For this review, take the finished solid that the model builds, in its own axes (mm). Coordinates: 2 decimals unless noted, no trailing zeros. Write each loop counter-clockwise with the first axis right and the second up, starting at its lowest first coordinate (ties: lowest second). Pieces come first, ordered by that corner, then holes.
1) We need section A-A on z = 289.5. Write out the cut boundary in (x, y).
2) To check wall thickness, follow line 1 along Z through (x, y) = (146.5, -148.5); line 2 along X through (y, z) = (301, 546); line 3 along X through (y, z) = (57, 558.5). State the ranges of each line that lie inside material, in increasing order.
3) Insertion check: P1, Ø25, axis at y = -366.5, z = 110.5, coming from the -X side; P2, Ø10, axis at x = -10, y = -285, coming from the -Z side; P3, Ø8, axis at x = -138.5, y = 116, coming from the +Z side. Each pin has a flat end and moves straight along its axis. Give the tip position at first contact, or say it passes through.
4) We need section C-C on y = -138. Write out the cut boundary in (x, z), then the cut area to 3 significant figures.
5) We need section B-B on y = 24. Write out the cut boundary in (x, z), then the cut area to 3 significant figures.
6) We need section D-D on x = 92.5. Write out the cut boundary in (y, z).
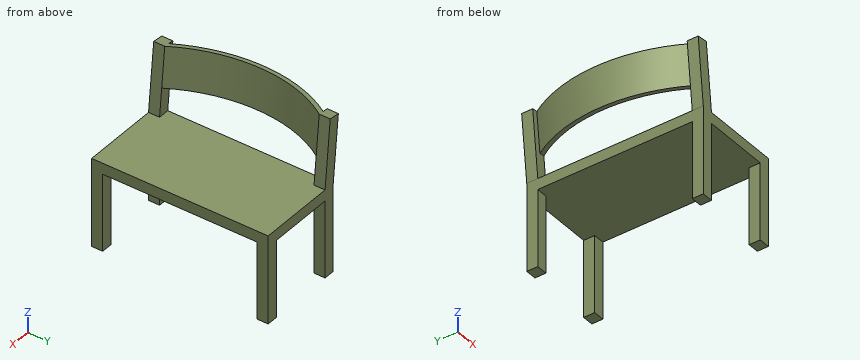
from build123d import *

# Parameters (mm, degrees)
F0_W       = 400
F0_H       = 800
F1_DEPTH   = 400
F2_W       = 300
F2_H       = 350
F3_DEPTH   = 800.001
F4_W       = 700
F4_H       = 350
F5_DEPTH   = 400.001
F10_W      = 800
F10_H      = 300
F11_DEPTH  = 50
F12_W      = 700
F12_H      = 300
F13_DEPTH  = 429.5428217516
F13_FACE_W = 50
F13_FACE_H = 50
F18_DEPTH  = 180


with BuildPart() as f1:
    # F0 (on Top) → F1 (new body)
    with BuildSketch(Plane.XY):
        Rectangle(F0_W, F0_H)
    extrude(amount=F1_DEPTH)

    # F2 (on face) → F3 (cut, through all)
    with BuildSketch(Plane.XZ.offset(400)):
        with Locations((0, 175)):
            Rectangle(F2_W, F2_H)
    extrude(amount=-F3_DEPTH, mode=Mode.SUBTRACT)

    # F4 (on face) → F5 (cut, through all)
    with BuildSketch(Plane.YZ.offset(200)):
        with Locations((0, 175)):
            Rectangle(F4_W, F4_H)
    extrude(amount=-F5_DEPTH, mode=Mode.SUBTRACT)

    # F10 (on face) → F11 (join)
    with BuildSketch(Plane(origin=(-156.2324219098, 0, -16.4206892285), x_dir=(0, 1, 0), z_dir=(0.9945218954, 0, 0.1045284633))):
        with Locations((0, 568.7144508008)):
            Rectangle(F10_W, F10_H)
    extrude(amount=F11_DEPTH)

    # F12 (on face) → F13 (cut, through all)
    with BuildSketch(Plane(origin=(-156.2324219098, 0, -16.4206892285), x_dir=(0, -1, 0), z_dir=(-0.9945218954, 0, -0.1045284633))):
        with Locations((0, 568.7144508008)):
            Rectangle(F12_W, F12_H)
    extrude(amount=-F13_DEPTH, mode=Mode.SUBTRACT)

    # F13_face (on face) → F14 (join, up to the next surface of F1)
    with BuildSketch(Plane(origin=(-175.1369526158, -375, 402.6132115817), x_dir=(1, 0, 0), z_dir=(0.1045284633, 0, -0.9945218954))):
        Rectangle(F13_FACE_W, F13_FACE_H)
    extrude(until=Until.NEXT)

    # F13_face (on face) → F15 (join, up to the next surface of F1)
    with BuildSketch(Plane(origin=(-175.1369526158, -375, 402.6132115817), x_dir=(1, 0, 0), z_dir=(0.1045284633, 0, -0.9945218954))):
        with Locations((0, -750)):
            Rectangle(F13_FACE_W, F13_FACE_H)
    extrude(until=Until.NEXT)

    # F17 (on plane+point) → F18 (join)
    with BuildSketch(Plane(origin=(-75.1261170705, 0, 714.777257839), x_dir=(0.9945218954, 0, 0.1045284633), z_dir=(-0.1045284633, 0, 0.9945218954))):
        with BuildLine():
            ThreePointArc((-107.0929937666, -350), (-219.7532765261, 0), (-107.0929937666, 350))
            Line((-107.0929937666, 350), (-123.3376510079, 361.6666666667))
            ThreePointArc((-123.3376510079, 361.6666666667), (-239.7532765261, 0), (-123.3376510079, -361.6666666667))
            Line((-123.3376510079, -361.6666666667), (-107.0929937666, -350))
        make_face()
    extrude(amount=-F18_DEPTH)


solid = f1.part
Result:
1. outline: (-200, -400) - (-150, -400) - (-150, -350) - (-200, -350) - close; (-200, 350) - (-150, 350) - (-150, 400) - (-200, 400) - close; (150, -400) - (200, -400) - (200, -350) - (150, -350) - close; (150, 350) - (200, 350) - (200, 400) - (150, 400) - close
2. line 1: z = 350 to 400
2. line 2: x = -220.06 to -196.94
2. line 3: x = -297.13 to -276.94
3. P1: stops at x = -200
3. P2: stops at z = 350
3. P3: stops at z = 400
4. outline: (-298.1, 691.34) - (-279.28, 512.33) - (-258.86, 514.47) - (-277.68, 693.49) - close; (-200, 350) - (200, 350) - (200, 400) - (-200, 400) - close
4. area: 23,700 mm2
5. outline: (-313.1, 689.76) - (-294.29, 510.75) - (-274.38, 512.84) - (-293.2, 691.86) - close; (-200, 350) - (200, 350) - (200, 400) - (-200, 400) - close
5. area: 23,600 mm2
6. outline: (-400, 350) - (400, 350) - (400, 400) - (-400, 400) - close
